Check sheet for the modelled part. Datum: model origin and axes. Units: mm. A direction names the side the tool comes from. Coordinates: 2 decimals unless noted, no trailing zeros. Loops run counter-clockwise (first coordinate to the right, second up) from the corner with the lowest first, then second, coordinate; pieces in that order, holes last.
Autodesk Inventor part; units mm, degrees
ref_plane "YZ Plane" through (0, 0, 0) normal (1, 0, 0) x (0, 1, 0)
ref_plane "XZ Plane" through (0, 0, 0) normal (0, 1, 0) x (-1, 0, 0)
ref_plane "XY Plane" through (0, 0, 0) normal (0, 0, 1) x (1, 0, 0)
sketch "Sketch1" plane through (0, 0, 0) normal (0, 1, 0) x (-1, 0, 0)
  arc A0 (2.1415, -16.469) -> (0, -13.652) centre (0, -15.8745) ccw
  line L0 (7.0734, 0) -> (7.0734, -9.8745)
  line L1 (0, 0.4443) -> (0, -21.7427) construction
  line L2 (-7.0734, 0) -> (-7.0734, -9.8745)
  arc A1 (0, -13.652) -> (-2.1415, -16.469) centre (0, -15.8745) ccw
  line L3 (4, -22.8384) -> (4, -25.8745)
  line L4 (-4, -22.8384) -> (-4, -25.8745)
  arc A2 (2, -25.8745) -> (4, -25.8745) centre (3, -25.8745) ccw
  arc A3 (-4, -25.8745) -> (-2, -25.8745) centre (-3, -25.8745) ccw
  line L5 (3.0734, 0) -> (3.0734, -9.652)
  line L6 (3.0734, -9.652) -> (-3.0734, -9.652)
  line L7 (-3.0734, -9.652) -> (-3.0734, 0)
  line L8 (7.0734, 0) -> (3.0734, 0)
  line L9 (-3.0734, 0) -> (-7.0734, 0)
  spline S0 degree 4 poles (2, -25.8745) (2, -23.2445) (1.6155, -19.943) (1.6024, -18.411) (2.1415, -16.469) knots 0 0 0 0 0 1 1 1 1 1
  spline S1 degree 4 poles (-2, -25.8745) (-2, -23.2445) (-1.6155, -19.943) (-1.6024, -18.411) (-2.1415, -16.469) knots 0 0 0 0 0 1 1 1 1 1
  spline S2 degree 4 poles (7.0734, -9.8745) (7.0734, -11.5508) (4.5976, -10.8217) (4, -18.7622) (4, -22.8384) knots 0 0 0 0 0 1 1 1 1 1
  spline S3 degree 4 poles (-7.0734, -9.8745) (-7.0734, -11.5508) (-4.5976, -10.8217) (-4, -18.7622) (-4, -22.8384) knots 0 0 0 0 0 1 1 1 1 1
  point P0 (0, 0)
  point P1 (0, -9.652)
  point P2 (1.75, -19.9116)
  point P3 (-1.75, -19.9116)
  point P4 (6.2466, -11.4624)
  point P5 (-6.2466, -11.4624)
  dimension "d6" = 6
  dimension "d7" = 1
  dimension "d8" = 2.2225
  dimension "d19" = 9.652
  dimension "d20" = 6.1468
  dimension "d27" = 4
  dimension "d31" = 4
  dimension "d34" = 3.5
  dimension "d35" = 10
  dimension "d37" = 4
extrude "Extrusion1" add sketch "Sketch1" along normal blind 10
sketch "Sketch2" plane through (7.0734, 0, 0) normal (1, 0, 0) x (0, 0, -1)
  circle A0 centre (5.08, 5) radius 2.2225
  line L0 (0, 10) -> (9.8745, 10)
  line L1 (0, 0) -> (0, 10)
  point P0 (9.652, 10)
  dimension "d14" = 4.445
  dimension "d15" = 5
  dimension "d32" = 4.572
extrude "Extrusion2" cut sketch "Sketch2" against normal blind 15
sketch "Sketch3" plane through (4, 0, -22.8384) normal (1, 0, 0) x (0, 0, -1)
  circle A0 centre (-17.7584, 5) radius 2.2225
  line L0 (3.0361, 0) -> (3.0361, 10)
  line L1 (0.0361, 5) -> (1.518, 10) construction
  line L2 (3.0361, 10) -> (0, 10) construction
  line L3 (0.5361, 5) -> (-0.4639, 5) construction
  line L4 (0.5361, 6.651) -> (-0.4639, 6.651)
  line L5 (-0.4639, 3.349) -> (0.5361, 3.349)
  arc A1 (0.5361, 3.349) -> (0.5361, 6.651) centre (0.5361, 5) ccw
  arc A2 (-0.4639, 6.651) -> (-0.4639, 3.349) centre (-0.4639, 5) ccw
  point P0 (-22.8384, 0)
  dimension "d21" = 3
  dimension "d24" = 1
  dimension "d30" = 1.651
extrude "Extrusion3" cut sketch "Sketch3" along normal mid plane 20 contours A1 L5 A2 L4
sketch "Sketch4" plane through (-7.0734, 0, -9.8745) normal (-1, 0, 0) x (0, 0, 1)
  line L0 (0, 0) -> (9.8745, 0)
  line L1 (9.8745, 0) -> (9.8745, 10)
  line L2 (0, 10) -> (9.8745, 10)
  line L3 (0, 0) -> (0, 10)
  circle A0 centre (4.7945, 5) radius 2.2225
  line L4 (6.9209, 8.683) -> (9.0473, 5)
  line L5 (9.0473, 5) -> (6.9209, 1.317)
  line L6 (6.9209, 1.317) -> (2.6681, 1.317)
  line L7 (2.6681, 1.317) -> (0.5417, 5)
  line L8 (0.5417, 5) -> (2.6681, 8.683)
  line L9 (2.6681, 8.683) -> (6.9209, 8.683)
  dimension "d25" = 7.366
extrude "Extrusion4" cut sketch "Sketch4" against normal blind 1.27 contours A0 | L4 L5 L6 L7 L8 L9
sketch "Sketch5" plane through (-4, 0, -25.8745) normal (-1, 0, 0) x (0, 0, 1)
  line L0 (1.3496, 7.921) -> (4.7225, 7.921)
  line L1 (4.7225, 7.921) -> (6.4089, 5)
  line L2 (6.4089, 5) -> (4.7225, 2.079)
  line L3 (4.7225, 2.079) -> (1.3496, 2.079)
  line L4 (1.3496, 2.079) -> (-0.3368, 5)
  line L5 (-0.3368, 5) -> (1.3496, 7.921)
  arc A0 (2.5, 6.651) -> (2.5, 3.349) centre (2.5, 5) ccw
  point P0 (25.8745, 0)
  point P1 (3.0361, 5)
  point P2 (3.5, 6.651)
  point P3 (3.5, 3.349)
  point P4 (3.0361, 6.651)
  point P5 (3.0361, 3.349)
  dimension "d38" = 5.842
extrude "Extrusion5" cut sketch "Sketch5" along normal mid plane 2.54
sketch "Sketch6" plane through (-3.0734, 0, 0) normal (1, 0, 0) x (0, 0, -1)
  line L0 (9.652, 0) -> (0, 0)
  line L1 (9.652, 10) -> (0, 10)
  arc A0 (8.9662, 0) -> (8.9662, 10) centre (-8.9178, 5) ccw
  line L2 (0, 10) -> (9.8745, 10)
  line L3 (9.8745, 0) -> (9.8745, 10)
  line L4 (0, 0) -> (9.8745, 0)
  line L5 (9.652, 0) -> (9.652, 10)
  point P0 (9.652, 5)
  point P1 (9.652, 4.8706)
  dimension "d41" = 0.6858
  dimension "d44" = 0.6858
extrude "Extrusion6" add sketch "Sketch6" along normal blind 10
equation "\"TUBE\" = 4.445"
equation "\"SCREW\" = 3.302"
equation "\"HEX\" = 5.842"
equation "\"HEX_DEPTH\" = 1.27"
properties part number "SlideClip"
1) Section check B-B on z = -1.75. Enter the section's corners in (x, y), plus the area to 3 significant figures.
Answer sheet:
outline: (-7.07, 0) - (-3.07, 0) - (-3.07, 10) - (-7.07, 10) - (-7.07, 6.6) - (-5.8, 6.6) - (-5.8, 3.4) - (-7.07, 3.4) - close; (3.07, 0) - (7.07, 0) - (7.07, 10) - (3.07, 10) - close
area: 75.9 mm2
2) Section check A-A on z = -5.08. Enter the section's corners in (x, y).
Answer sheet:
outline: (-7.07, 0) - (-3.07, 0) - (-3.07, 2.78) - (-5.8, 2.78) - (-5.8, 1.32) - (-7.07, 1.32) - close; (-7.07, 8.68) - (-5.8, 8.68) - (-5.8, 7.22) - (-3.07, 7.22) - (-3.07, 10) - (-7.07, 10) - close; (3.07, 0) - (7.07, 0) - (7.07, 2.78) - (3.07, 2.78) - close; (3.07, 7.22) - (7.07, 7.22) - (7.07, 10) - (3.07, 10) - close
3) Set-up check for faces 5 (the cylindrical face through (-1.752, 4.93, -14.507)), 6 (the flat face through (-6.45, 3.18, -1.88)), 7 (the flat face through (-2.3, 3.349, -22.9)): record each of +Z, -Z, +X, -X, +Y, -Y from which the full face is reachable in a straight line by a thin tool's end or side.
Answer sheet:
face 5: +Y, -Y
face 6: -X
face 7: +X, -X
4) Depth check by flat-ended pin: pin 1 (0.7 mm diameter, centred on x = -3.5, z = -23, fed in from -Y); pin 2 (1.5 mm diameter, centred on y = 7.5, z = -24.5, fed in from -X); pin 3 (1 mm diameter, centred on y = 8, z = -10.5, fed in from +X); pin 4 (3 mm diameter, centred on y = 6.5, z = -3.5, fed in from -X). Enter the tip coordinate at first touch or a pass-through.
Answer sheet:
pin 1: stops at y = 0
pin 2: stops at x = -4
pin 3: stops at x = 7.07
pin 4: stops at x = -5.8
5) Scan lines: line 1 (Y direction, x = 4.9, z = -5.08); line 2 (X direction, y = 7.75, z = -8.75); line 3 (X direction, y = 3.75, z = -3). Record each from-to range of solid material in increasing order.
Answer sheet:
line 1: y = 0 to 2.78, 7.22 to 10
line 2: x = -7.07 to -3.07, 3.07 to 7.07
line 3: x = -5.8 to -3.07, 3.07 to 7.07
6) Mould release check, pull along Z, two halves, no side actions. Record for faces 1 (the flat face through (0, 0, -10)), 2 (the flat face through (-3.36, 6.44, -25.38)), 3 (the flat face through (-5, 5, 0)), 4 (the flat face through (-3, 2.079, -23)): +Z half, -Z half, draft (parallel to the pull), parting line (faces both ways), or undercut.
Answer sheet:
face 1: draft
face 2: undercut
face 3: +Z half
face 4: undercut
